from build123d import *

# Parameters (mm, degrees)
IZIM1_W                     = 96.5
IZIM1_H                     = 40.6
Y_KSEKLIK_EKSTR_ZYON1_DEPTH = 110
KES_EKSTR_ZYON1_DEPTH       = 92.5
IZIM3_W                     = 92.5
IZIM3_H                     = 36.6
KES_EKSTR_ZYON2_DEPTH       = 2
IZIM4_W                     = 86.5
IZIM4_H                     = 30.6
KES_EKSTR_ZYON3_DEPTH       = 13.5
RADYUS1_R                   = 2
RADYUS2_R                   = 1
IZIM5_W                     = 20
IZIM5_H                     = 5
KES_EKSTR_ZYON4_DEPTH       = 3.5
IZIM6_W                     = 9.1
IZIM6_H                     = 3.15
KES_EKSTR_ZYON5_DEPTH       = 1.5
IZIM7_W                     = 1
IZIM7_H                     = 23.6
KES_EKSTR_ZYON6_DEPTH       = 2


with BuildPart() as part:
    # Çizim1 → Yükseklik-Ekstrüzyon1 (new body)
    with BuildSketch(Plane.XY):
        Rectangle(IZIM1_W, IZIM1_H)
    extrude(amount=Y_KSEKLIK_EKSTR_ZYON1_DEPTH)

    # Çizim2 → Kes-Ekstrüzyon1 (cut)
    with BuildSketch(Plane.XY.offset(110)):
        Polygon((-46.25, -18.3), (-42.75, -18.3), (-42.75, -20.3), (42.75, -20.3), (42.75, -18.3), (46.25, -18.3), (46.25, 18.3), (42.75, 18.3), (42.75, 20.3), (-42.75, 20.3), (-42.75, 18.3), (-46.25, 18.3), align=None)
    extrude(amount=-KES_EKSTR_ZYON1_DEPTH, mode=Mode.SUBTRACT)

    # Çizim3 → Kes-Ekstrüzyon2 (cut)
    with BuildSketch(Plane.XY.offset(17.5)):
        Rectangle(IZIM3_W, IZIM3_H)
    extrude(amount=-KES_EKSTR_ZYON2_DEPTH, mode=Mode.SUBTRACT)

    # Çizim4 → Kes-Ekstrüzyon3 (cut)
    with BuildSketch(Plane.XY.offset(15.5)):
        Rectangle(IZIM4_W, IZIM4_H)
    extrude(amount=-KES_EKSTR_ZYON3_DEPTH, mode=Mode.SUBTRACT)

    # Radyus1
    radyus1_edges = [part.edges().sort_by_distance(p)[0] for p in [
        (42.75, -19.3, 17.5),
        (-42.75, -19.3, 17.5),
        (-42.75, 19.3, 17.5),
        (42.75, 19.3, 17.5),
        (0, -20.3, 0),
        (-48.25, 0, 0),
        (0, 20.3, 0),
        (48.25, 0, 0),
        (43.25, 15.3, 8.75),
        (43.25, -15.3, 8.75),
        (-43.25, -15.3, 8.75),
        (-43.25, 15.3, 8.75),
        (48.25, -20.3, 55),
        (-48.25, -20.3, 55),
        (-48.25, 20.3, 55),
        (48.25, 20.3, 55),
    ]]
    fillet(radyus1_edges, radius=RADYUS1_R)

    # Radyus2
    radyus2_edges = [part.edges().sort_by_distance(p)[0] for p in [
        (46.25, 18.3, 62.75),
        (46.25, -18.3, 62.75),
        (-46.25, -18.3, 62.75),
        (-46.25, 18.3, 62.75),
    ]]
    fillet(radyus2_edges, radius=RADYUS2_R)

    # Çizim5 → Kes-Ekstrüzyon4 (cut)
    with BuildSketch(Plane.XZ.offset(-15.3)):
        with Locations((27.75, 4.5)):
            Rectangle(IZIM5_W, IZIM5_H)
    extrude(amount=-KES_EKSTR_ZYON4_DEPTH, mode=Mode.SUBTRACT)

    # Pah3
    # the kernel refuses this chamfer: 8.5, 5 mm, written as the material it takes off along each edge
    with BuildSketch(Plane(origin=(37.75, 15.3, 7), x_dir=(0, -0.01960111388009259, 0.9998078797122274), z_dir=(-1, 0, 0))) as pah3_piece_1_section:
        with BuildLine():
            Line((8.794747283, 0), (-0.394385874, 5.165648867))
            Line((-0.394385874, 5.165648867), (-0.564353214, 5.162316677))
            ThreePointArc((-0.564353214, 5.162316677), (-0.220659611, 2.582364372), (-0.16996734, -0.003332189))
            Line((-0.16996734, -0.003332189), (0.003332189, -0.16996734))
            ThreePointArc((0.003332189, -0.16996734), (4.399016344, -0.083790478), (8.798079472, -0.16996734))
            Line((8.798079472, -0.16996734), (8.794747283, 0))
        make_face()
    pah3_piece_1 = extrude(amount=20, mode=Mode.PRIVATE)
    pah3_piece_1 = split(pah3_piece_1, bisect_by=Plane(origin=(27.75, 18.8, 10.101795291), z_dir=(0, -1, 0)), keep=Keep.TOP, mode=Mode.PRIVATE)
    add(pah3_piece_1, mode=Mode.SUBTRACT)

    # Çizim6 → Kes-Ekstrüzyon5 (cut)
    with BuildSketch(Plane.XZ.offset(-18.8)):
        with Locations((27.75, 4.625)):
            Rectangle(IZIM6_W, IZIM6_H)
    extrude(amount=-KES_EKSTR_ZYON5_DEPTH, mode=Mode.SUBTRACT)

    # Çizim7 → Kes-Ekstrüzyon6 (cut)
    with BuildSketch(Plane.XY.offset(2)):
        with Locations((17.75, 0)):
            Rectangle(IZIM7_W, IZIM7_H)
        with Locations((14.75, 0)):
            Rectangle(IZIM7_W, IZIM7_H)
        with Locations((11.75, 0)):
            Rectangle(IZIM7_W, IZIM7_H)
        with Locations((8.75, 0)):
            Rectangle(IZIM7_W, IZIM7_H)
        with Locations((5.75, 0)):
            Rectangle(IZIM7_W, IZIM7_H)
        with Locations((2.75, 0)):
            Rectangle(IZIM7_W, IZIM7_H)
        with Locations((-0.25, 0)):
            Rectangle(IZIM7_W, IZIM7_H)
        with Locations((-3.25, 0)):
            Rectangle(IZIM7_W, IZIM7_H)
        with Locations((-6.25, 0)):
            Rectangle(IZIM7_W, IZIM7_H)
        with Locations((-9.25, 0)):
            Rectangle(IZIM7_W, IZIM7_H)
        with Locations((-12.25, 0)):
            Rectangle(IZIM7_W, IZIM7_H)
        with Locations((-15.25, 0)):
            Rectangle(IZIM7_W, IZIM7_H)
    extrude(amount=-KES_EKSTR_ZYON6_DEPTH, mode=Mode.SUBTRACT)


solid = part.part
Part model, mm, in its own coordinate system. A direction names the side the tool comes from. Round coordinates to 2 decimals unless told otherwise and drop trailing zeros. Order: outer loops, then holes, each group sorted by start corner. A loop starts at its lowest first (then second) coordinate and runs counter-clockwise, first axis right, second up. Notation, with made-up numbers: (68, 13) -> (97, 13) arc R12 ccw to (97, 33) -> close; hole circle Ø3 at (-7, 78.25). An arc over 180 degrees is marked (long way). Put each result on its own line as item: value.
Q1. Band-saw the part on C-C (y = 8.5). State how many separate pieces and enclosed holes the cut face has, and give its area (3 significant figures).
From the geometry:
separate pieces: 13
enclosed holes: 0
area: 680 mm2
Q2. Band-saw the part on D-D (x = 35). Give the cut face in (y, z), and give its area (3 significant figures).
From the geometry:
outline: (-20.3, 2) arc R2 ccw to (-18.3, 0) -> (18.3, 0) arc R2 ccw to (20.3, 2) -> (20.3, 17.5) -> (18.3, 17.5) -> (18.3, 15.5) -> (15.3, 15.5) -> (18.8, 9.55) -> (18.8, 2) -> (-15.3, 2) -> (-15.3, 15.5) -> (-18.3, 15.5) -> (-18.3, 17.5) -> (-20.3, 17.5) -> close
area: 186 mm2
Q3. Band-saw the part on B-B (x = -39.5). Give the cut face in (y, z), and give its area (3 significant figures).
From the geometry:
outline: (-20.3, 2) arc R2 ccw to (-18.3, 0) -> (18.3, 0) arc R2 ccw to (20.3, 2) -> (20.3, 17.5) -> (18.3, 17.5) -> (18.3, 15.5) -> (15.3, 15.5) -> (15.3, 2) -> (-15.3, 2) -> (-15.3, 15.5) -> (-18.3, 15.5) -> (-18.3, 17.5) -> (-20.3, 17.5) -> close
area: 222 mm2
Q4. Band-saw the part on A-A (z = 70.5). Give the cut face in (x, y), and give its area (3 significant figures).
From the geometry:
outline: (-48.25, -18.3) arc R2 ccw to (-46.25, -20.3) -> (-42.75, -20.3) -> (-42.75, -18.3) -> (-45.25, -18.3) arc R1 cw to (-46.25, -17.3) -> (-46.25, 17.3) arc R1 cw to (-45.25, 18.3) -> (-42.75, 18.3) -> (-42.75, 20.3) -> (-46.25, 20.3) arc R2 ccw to (-48.25, 18.3) -> close; (42.75, -20.3) -> (46.25, -20.3) arc R2 ccw to (48.25, -18.3) -> (48.25, 18.3) arc R2 ccw to (46.25, 20.3) -> (42.75, 20.3) -> (42.75, 18.3) -> (45.25, 18.3) arc R1 cw to (46.25, 17.3) -> (46.25, -17.3) arc R1 cw to (45.25, -18.3) -> (42.75, -18.3) -> close
area: 188 mm2
Q5. Pull direction X, two halves, no side cores. Call faces 4 (the face through (0, -20.3, 16)), 5 (the face through (-48.25, 0, 55)), 6 (the face through (27.89, 17.026, 12.567)): pulls with the +X half, pulls with the -X half, needs draft (parallel to the pull), parting line crosses it, or undercut.
From the geometry:
face 4: needs draft
face 5: pulls with the -X half
face 6: undercut
Q6. Wall check: line 1 (Y direction, x = 43, z = 27); line 2 (X direction, y = 4.5, z = 26); line 3 (Y direction, x = -4.5, z = 8.5). Give the ranges that are in metal, low to high. Write a range as [from, to].
From the geometry:
line 1: y = [-20.3, -18.3], [18.3, 20.3]
line 2: x = [-48.25, -46.25], [46.25, 48.25]
line 3: y = [-20.3, -15.3], [15.3, 20.3]
Q7. Tool access for faces 1 (the face through (48.25, 0, 55)), 2 (the face through (28, 18.8, 7)), 3 (the face through (46.25, 0, 63)): list every direction of +Z, -Z, +X, -X, +Y, -Y with a clear straight run to the whole face (end or side of a thin tool).
From the geometry:
face 1: +Z, -Z, +X, +Y, -Y
face 2: none
face 3: +Z
Q8. Pin check, flat tips, straight feed: pin 1 Ø1.1 at (x, z) = (-12, 1) entering from -Y; pin 2 Ø0.5 at (x, z) = (9, 0.5) entering from -Y; pin 3 Ø8 at (x, y) = (17, 16) entering from +Z; pin 4 Ø2 at (y, z) = (0, 1) entering from -X. Stop position of each tip, or through.
From the geometry:
pin 1: stops at y = -20.25
pin 2: stops at y = -19.86
pin 3: stops at z = 17.5
pin 4: stops at x = -48.25
